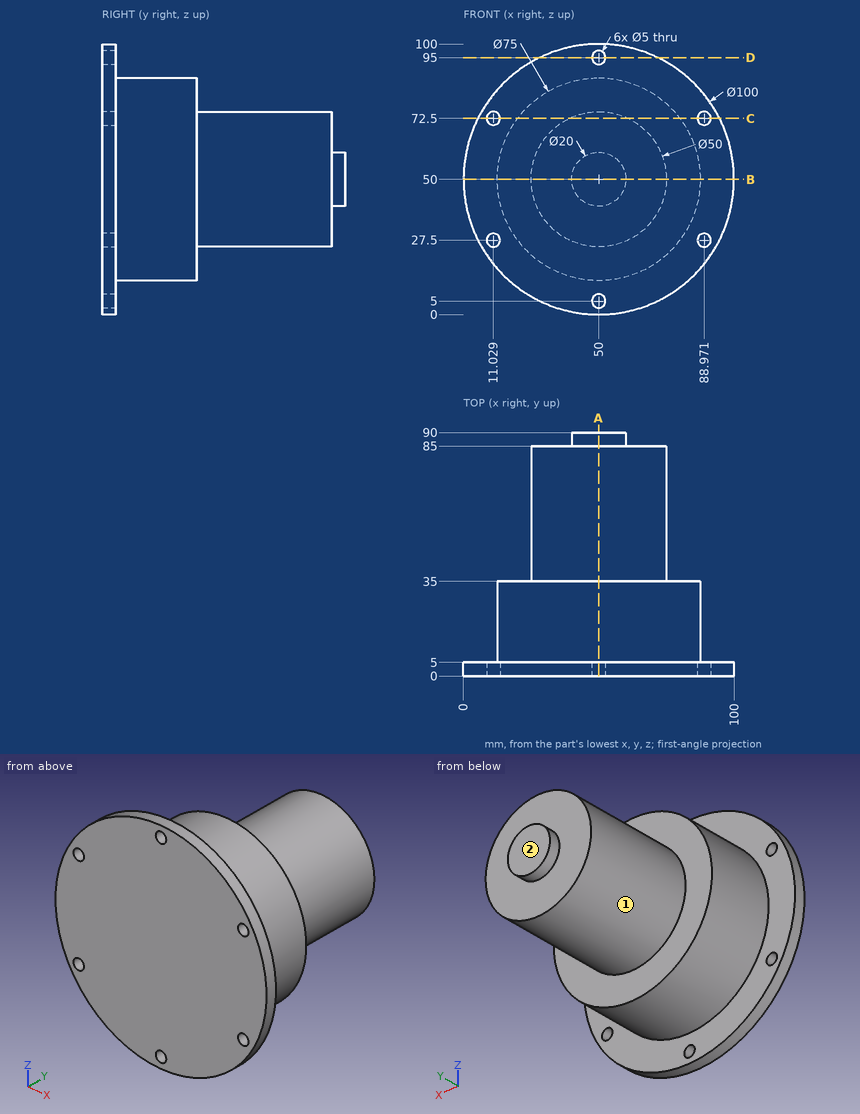
For this review, use the dimensioned drawing (mm, ordinates from the lowest corner) and the shaded views. A direction names the side the tool comes from. Give positions to 0.01 mm unless a question says otherwise; leave off trailing zeros. Write each loop counter-clockwise with the first axis right and the second up, starting at its lowest first coordinate (ties: lowest second). Pieces come first, ordered by that corner, then holes.
(1) Tool access review of the marked faces 1 and 2: name each direction out of +Z, -Z, +X, -X, +Y, -Y from which nothing blocks a thin tool from reaching the whole face with its end or side.
(2) For P1, Ø8, axis at x = 79, y = 34, coming from the +Z side; P2, Ø2, axis at x = 69, y = 47.5, coming from the +Z side; P3, Ø5, axis at y = 55, z = 25.5, coming from the +X side (1 decimal), all flat-tipped, find the tip position at first contact; note any pin that passes through.
(3) Consider section D-D, the plane z = 95. Give the boundary of the cut face in (x, y).
(4) Consider section C-C, the plane z = 72.5. Give the boundary of the cut face in (x, y), and give its area (3 significant figures).
(5) Consider section B-B, the plane z = 50. Give the boundary of the cut face in (x, y).
(6) To check wall thickness, follow L1, parallel to X at y = 1.35, z = 72.5; L2, parallel to Y at x = 75.5, z = 27; L3, parallel to Y at x = 28, z = 87. State the ranges of each line that lie inside material, in increasing order.
(7) Consider section A-A, the plane x = 50. Give the boundary of the cut face in (y, z), and give its area (3 significant figures).
Returned:
1. face 1: +Y
1. face 2: +Z, -Z, +X, -X, +Y
2. P1: stops at z = 77.95
2. P2: stops at z = 67.35
2. P3: stops at x = 61.9
3. outline: (28.21, 0) - (47.5, 0) - (47.5, 5) - (28.21, 5) - close; (52.5, 0) - (71.79, 0) - (71.79, 5) - (52.5, 5) - close
4. outline: (5.35, 0) - (8.53, 0) - (8.53, 5) - (5.35, 5) - close; (13.53, 0) - (86.47, 0) - (86.47, 5) - (80, 5) - (80, 35) - (60.9, 35) - (60.9, 85) - (39.1, 85) - (39.1, 35) - (20, 35) - (20, 5) - (13.53, 5) - close; (91.47, 0) - (94.65, 0) - (94.65, 5) - (91.47, 5) - close
4. area: 3,290 mm2
5. outline: (0, 0) - (100, 0) - (100, 5) - (87.5, 5) - (87.5, 35) - (75, 35) - (75, 85) - (60, 85) - (60, 90) - (40, 90) - (40, 85) - (25, 85) - (25, 35) - (12.5, 35) - (12.5, 5) - (0, 5) - close
6. L1: x = 5.35 to 8.53, 13.53 to 86.47, 91.47 to 94.65
6. L2: y = 0 to 35
6. L3: y = 0 to 5
7. outline: (0, 0) - (5, 0) - (5, 2.5) - (0, 2.5) - close; (0, 7.5) - (5, 7.5) - (5, 12.5) - (35, 12.5) - (35, 25) - (85, 25) - (85, 40) - (90, 40) - (90, 60) - (85, 60) - (85, 75) - (35, 75) - (35, 87.5) - (5, 87.5) - (5, 92.5) - (0, 92.5) - close; (0, 97.5) - (5, 97.5) - (5, 100) - (0, 100) - close
7. area: 5,300 mm2
